```python
from build123d import *

# Parameters (mm, degrees)
F0_W     = 585
F0_H     = 620
F1_DEPTH = 18
F2_W     = 585
F2_H     = 18
F3_DEPTH = 42
F4_W     = 21
F4_H     = 18
F5_DEPTH = 60


with BuildPart() as f1:
    # F0 (on Top) → F1 (new body)
    with BuildSketch(Plane.XY):
        Rectangle(F0_W, F0_H)
    extrude(amount=F1_DEPTH)

    # F2 (on face) → F3 (join)
    with BuildSketch(Plane(origin=(0, 0, 0), x_dir=(1, 0, 0), z_dir=(0, 0, -1))):
        with Locations((0, 301)):
            Rectangle(F2_W, F2_H)
    extrude(amount=F3_DEPTH)

    # F4 (on face) → F5 (cut)
    with BuildSketch(Plane.XY.offset(18)):
        with Locations((282, -301)):
            Rectangle(F4_W, F4_H)
    extrude(amount=-F5_DEPTH, mode=Mode.SUBTRACT)


solid = f1.part
```
Work out the finished part from the listing and answer in its coordinate system (mm). A direction names the side the tool comes from. Give positions to 0.01 mm unless a question says otherwise; leave off trailing zeros. Order: outer loops, then holes, each group sorted by start corner. A loop starts at its lowest first (then second) coordinate and runs counter-clockwise, first axis right, second up. Notation, with made-up numbers: (34.5, 42) - (85.5, 42) arc R7 ccw to (85.5, 53) - close; hole circle Ø10 at (83.5, 47.5). An arc over 180 degrees is marked (long way). One line per item, written item: value. Start each with the question number.
1. Section C-C, the plane y = 90.5 is taken. Write down the section's boundary in (x, z).
2. Which of the six approach directions +Z, -Z, +X, -X, +Y, -Y give full straight-line access (tool end or side, diameter ignored) to faces 1 (the face through (282, -292, 9)), 2 (the face through (-4, 13, 0)), 3 (the face through (-14, -301, -42))?
3. Each of these flat-tipped pins is pushed along its axis until it touches: pin 1 Ø6 at (x, z) = (24, -11.5) entering from +Y; pin 2 Ø14.5 at (y, z) = (-302.5, -21.5) entering from +X; pin 3 Ø14.5 at (x, z) = (283.5, 13) entering from -Y. Where does it stop, or does it pass through?
4. Section A-A, the plane x = -42 is taken. Write down the section's boundary in (y, z).
5. Section B-B, the plane z = -29 is taken. Write down the section's boundary in (x, y), then the cut area to 3 significant figures.
6. Consider line 1 (Z direction, x = -211.5, y = -214); line 2 (Y direction, x = -46, z = -5.5). Determine where each line is inside the solid, lowest interval first.
Filled sheet:
1. outline: (-292.5, 0) - (292.5, 0) - (292.5, 18) - (-292.5, 18) - close
2. face 1: +Z, -Z, +X, -Y
2. face 2: -Z, +X, -X, +Y
2. face 3: -Z, +X, -X, +Y, -Y
3. pin 1: y = -292
3. pin 2: x = 271.5
3. pin 3: y = -292
4. outline: (-310, -42) - (-292, -42) - (-292, 0) - (310, 0) - (310, 18) - (-310, 18) - close
5. outline: (-292.5, -310) - (271.5, -310) - (271.5, -292) - (-292.5, -292) - close
5. area: 10,200 mm²
6. line 1: 0 to 18
6. line 2: -310 to -292
